from build123d import *

# Parameters (mm, degrees)
F0_R     = 9
F1_DEPTH = 10
F2_R     = 8.4
F3_DEPTH = 48.5
F6_DEPTH = 12.919


# Not quite as in the source:
# - a fillet or chamfer that OpenCascade refuses, or shapes differently, is made with other operations: its cross-section is extruded or revolved along the edge and cut away or added


with BuildPart() as f1:
    # F0 (on Right) → F1 (new body)
    with BuildSketch(Plane.YZ):
        Circle(F0_R)
    extrude(amount=F1_DEPTH)

    # F2 (on Right) → F3 (join)
    with BuildSketch(Plane.YZ):
        Circle(F2_R)
    extrude(amount=-F3_DEPTH)

    # F4: fillet of radius 1 on 1 edges, made by hand

    # F4_s1 → F4_t2 (revolve, cut)
    with BuildSketch(Plane.XY):
        with BuildLine():
            ThreePointArc((0.916515139, 9), (0.3687925815, 8.8366600265), (0, 8.4))
            Line((0, 8.4), (0, 9))
            Line((0, 9), (0.916515139, 9))
        make_face()
    revolve(axis=Axis((0, 0, 0), (1, 0, 0)), mode=Mode.SUBTRACT)

    # F5 (on face) → F6 (cut)
    with BuildSketch(Plane(origin=(-48.5, 0, 0), x_dir=(0, -1, 0), z_dir=(-1, 0, 0))):
        with BuildLine():
            Line((0.5, 7.4), (0.5, 8.3851058431))
            ThreePointArc((0.5, 8.3851058431), (0, 8.4), (-0.5, 8.3851058431))
            Line((-0.5, 8.3851058431), (-0.5, 7.4))
            Line((-0.5, 7.4), (0.5, 7.4))
        make_face()
        with BuildLine():
            Line((-2.3699176332, 7.0280502568), (-2.7469013185, 7.9381693826))
            ThreePointArc((-2.7469013185, 7.9381693826), (-3.2145408319, 7.7605880731), (-3.670780851, 7.5554859502))
            Line((-3.670780851, 7.5554859502), (-3.2937971658, 6.6453668244))
            Line((-3.2937971658, 6.6453668244), (-2.3699176332, 7.0280502568))
        make_face()
        with BuildLine():
            Line((-4.8790367902, 5.5861435714), (-5.575611812, 6.2827185932))
            ThreePointArc((-5.575611812, 6.2827185932), (-5.939696962, 5.939696962), (-6.2827185932, 5.575611812))
            Line((-6.2827185932, 5.575611812), (-5.5861435714, 4.8790367902))
            Line((-5.5861435714, 4.8790367902), (-4.8790367902, 5.5861435714))
        make_face()
        with BuildLine():
            Line((-6.6453668244, 3.2937971658), (-7.5554859502, 3.670780851))
            ThreePointArc((-7.5554859502, 3.670780851), (-7.7605880731, 3.2145408319), (-7.9381693826, 2.7469013185))
            Line((-7.9381693826, 2.7469013185), (-7.0280502568, 2.3699176332))
            Line((-7.0280502568, 2.3699176332), (-6.6453668244, 3.2937971658))
        make_face()
        with BuildLine():
            Line((-7.4, 0.5), (-8.3851058431, 0.5))
            ThreePointArc((-8.3851058431, 0.5), (-8.4, 0), (-8.3851058431, -0.5))
            Line((-8.3851058431, -0.5), (-7.4, -0.5))
            Line((-7.4, -0.5), (-7.4, 0.5))
        make_face()
        with BuildLine():
            Line((-7.0280502568, -2.3699176332), (-7.9381693826, -2.7469013185))
            ThreePointArc((-7.9381693826, -2.7469013185), (-7.7605880731, -3.2145408319), (-7.5554859502, -3.670780851))
            Line((-7.5554859502, -3.670780851), (-6.6453668244, -3.2937971658))
            Line((-6.6453668244, -3.2937971658), (-7.0280502568, -2.3699176332))
        make_face()
        with BuildLine():
            Line((-5.5861435714, -4.8790367902), (-6.2827185932, -5.575611812))
            ThreePointArc((-6.2827185932, -5.575611812), (-5.939696962, -5.939696962), (-5.575611812, -6.2827185932))
            Line((-5.575611812, -6.2827185932), (-4.8790367902, -5.5861435714))
            Line((-4.8790367902, -5.5861435714), (-5.5861435714, -4.8790367902))
        make_face()
        with BuildLine():
            Line((-3.2937971658, -6.6453668244), (-3.670780851, -7.5554859502))
            ThreePointArc((-3.670780851, -7.5554859502), (-3.2145408319, -7.7605880731), (-2.7469013185, -7.9381693826))
            Line((-2.7469013185, -7.9381693826), (-2.3699176332, -7.0280502568))
            Line((-2.3699176332, -7.0280502568), (-3.2937971658, -6.6453668244))
        make_face()
        with BuildLine():
            Line((-0.5, -7.4), (-0.5, -8.3851058431))
            ThreePointArc((-0.5, -8.3851058431), (0, -8.4), (0.5, -8.3851058431))
            Line((0.5, -8.3851058431), (0.5, -7.4))
            Line((0.5, -7.4), (-0.5, -7.4))
        make_face()
        with BuildLine():
            Line((2.3699176332, -7.0280502568), (2.7469013185, -7.9381693826))
            ThreePointArc((2.7469013185, -7.9381693826), (3.2145408319, -7.7605880731), (3.670780851, -7.5554859502))
            Line((3.670780851, -7.5554859502), (3.2937971658, -6.6453668244))
            Line((3.2937971658, -6.6453668244), (2.3699176332, -7.0280502568))
        make_face()
        with BuildLine():
            Line((4.8790367902, -5.5861435714), (5.575611812, -6.2827185932))
            ThreePointArc((5.575611812, -6.2827185932), (5.939696962, -5.939696962), (6.2827185932, -5.575611812))
            Line((6.2827185932, -5.575611812), (5.5861435714, -4.8790367902))
            Line((5.5861435714, -4.8790367902), (4.8790367902, -5.5861435714))
        make_face()
        with BuildLine():
            Line((6.6453668244, -3.2937971658), (7.5554859502, -3.670780851))
            ThreePointArc((7.5554859502, -3.670780851), (7.7605880731, -3.2145408319), (7.9381693826, -2.7469013185))
            Line((7.9381693826, -2.7469013185), (7.0280502568, -2.3699176332))
            Line((7.0280502568, -2.3699176332), (6.6453668244, -3.2937971658))
        make_face()
        with BuildLine():
            Line((7.4, -0.5), (8.3851058431, -0.5))
            ThreePointArc((8.3851058431, -0.5), (8.4, 0), (8.3851058431, 0.5))
            Line((8.3851058431, 0.5), (7.4, 0.5))
            Line((7.4, 0.5), (7.4, -0.5))
        make_face()
        with BuildLine():
            Line((7.0280502568, 2.3699176332), (7.9381693826, 2.7469013185))
            ThreePointArc((7.9381693826, 2.7469013185), (7.7605880731, 3.2145408319), (7.5554859502, 3.670780851))
            Line((7.5554859502, 3.670780851), (6.6453668244, 3.2937971658))
            Line((6.6453668244, 3.2937971658), (7.0280502568, 2.3699176332))
        make_face()
        with BuildLine():
            Line((5.5861435714, 4.8790367902), (6.2827185932, 5.575611812))
            ThreePointArc((6.2827185932, 5.575611812), (5.939696962, 5.939696962), (5.575611812, 6.2827185932))
            Line((5.575611812, 6.2827185932), (4.8790367902, 5.5861435714))
            Line((4.8790367902, 5.5861435714), (5.5861435714, 4.8790367902))
        make_face()
        with BuildLine():
            Line((3.2937971658, 6.6453668244), (3.670780851, 7.5554859502))
            ThreePointArc((3.670780851, 7.5554859502), (3.2145408319, 7.7605880731), (2.7469013185, 7.9381693826))
            Line((2.7469013185, 7.9381693826), (2.3699176332, 7.0280502568))
            Line((2.3699176332, 7.0280502568), (3.2937971658, 6.6453668244))
        make_face()
    extrude(amount=-F6_DEPTH, mode=Mode.SUBTRACT)


solid = f1.part
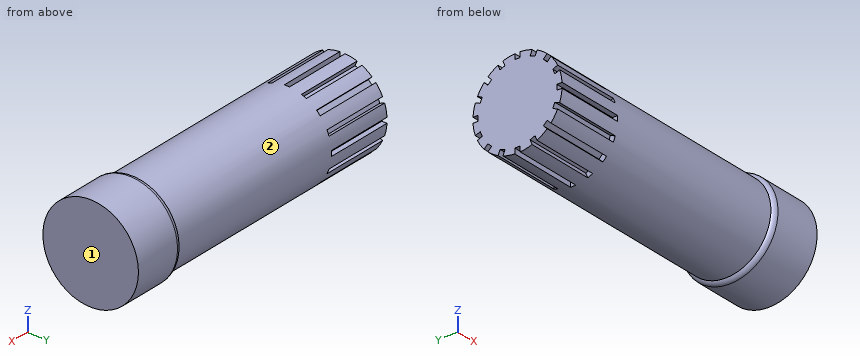
For this review, take the finished solid that the model builds, in its own axes (mm). Face numbers are marked on the shaded views. A direction names the side the tool comes from. Give positions to 0.01 mm unless a question says otherwise; leave off trailing zeros. Order: outer loops, then holes, each group sorted by start corner. A loop starts at its lowest first (then second) coordinate and runs counter-clockwise, first axis right, second up. Notation, with made-up numbers: (6, -39.5) -> (63, -39.5) arc R21 cw to (63, -30.5) -> close; hole circle Ø4 at (-34.75, -22.75). An arc over 180 degrees is marked (long way). Write item = value, one per line.
1) Insertion check: pin 1 (1 mm diameter, centred on x = -26, z = 6, fed in from +Y); pin 2 (1.1 mm diameter, centred on x = -40.5, y = 7.5, fed in from +Z); pin 3 (6 mm diameter, centred on x = -42.5, z = 3.5, fed in from +Y). Each pin has a flat end and moves straight along its axis. Give the tip position at first contact, or say it passes through.
Findings:
pin_1 = 6.35
pin_2 = 4.72
pin_3 = 8.39
2) We need section A-A, the plane x = -20. Give the boundary of the cut face in (y, z).
Findings:
outline = circle Ø16.8 at (0, 0)
3) To check wall thickness, follow L1, parallel to Y at x = -43, z = 5.25; L2, parallel to Y at x = -33.5, z = 2.75. State the ranges of each line that lie inside material, in increasing order. Write a range as from..to.
Findings:
L1 = -6.56..-5.96, -5.22..5.22, 5.96..6.56
L2 = -7.94..7.94
4) For the marked faces 1 and 2, list the 3-axis set-ups (+Z, -Z, +X, -X, +Y, -Y) from which the entire face can be reached by the end or side of a thin tool; tool diameter is ignored.
Findings:
face_1 = +Z, -Z, +X, +Y, -Y
face_2 = -X
